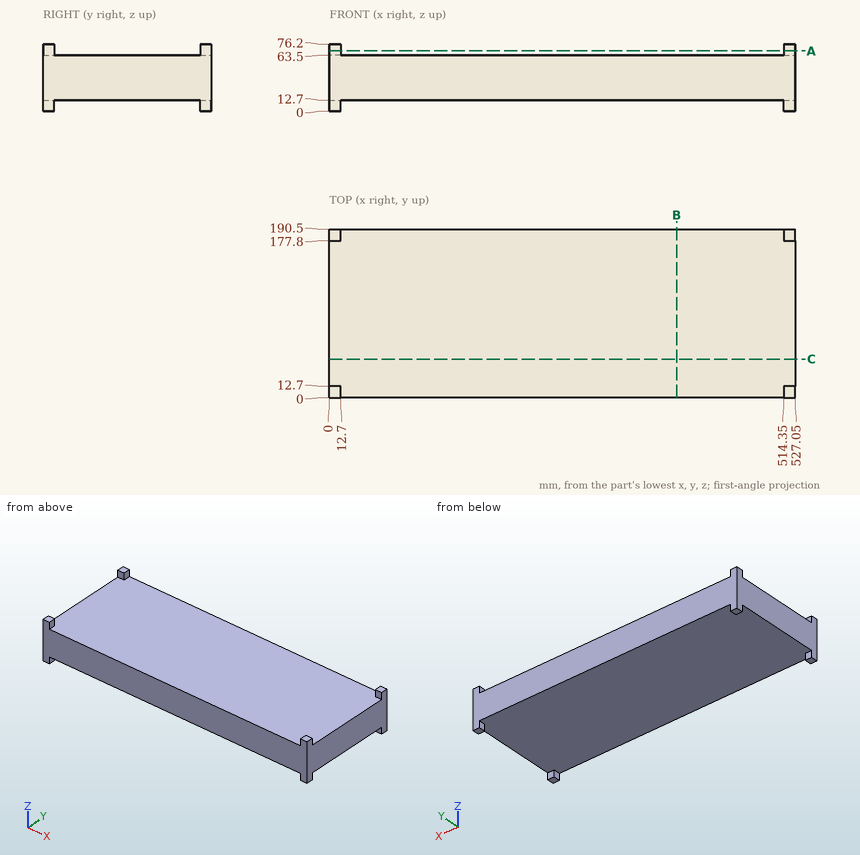
The figure shows three views and two pictorial views of one solid part (mm, origin at its lowest corner). Answer the questions. Round coordinates to 2 decimals unless told otherwise and drop trailing zeros. Write each loop counter-clockwise with the first axis right and the second up, starting at its lowest first coordinate (ties: lowest second). Pieces come first, ordered by that corner, then holes. Notation, with made-up numbers: M 76,65 L 134,65 A32 ccw 134,95 Z; hole C 85,39.25 d7. An arc over 180 degrees is marked long. Write each question's results on one line, items separated by ' | '. Start each with the question number.
(1) The part is cut by section C-C, the plane y = 43.5. Write down the section's boundary in (x, z).
(2) Each of these flat-tipped pins is pushed along its axis until it touches: P1, Ø8, axis at x = 93.5, y = 24.5, coming from the -Z side; P2, Ø1, axis at x = 90, y = 138.5, coming from the +Z side. Where does it stop, or does it pass through?
(3) The part is cut by section A-A, the plane z = 68.5. Write down the section's boundary in (x, y), and give its area (3 significant figures).
(4) The part is cut by section B-B, the plane x = 393. Write down the section's boundary in (y, z).
(5) Find the intervals of material crossed by line 1 (Z direction, x = 229, y = 169), in increasing order.
Worked answers:
1) outline: M 0,12.7 L 527.05,12.7 L 527.05,63.5 L 0,63.5 Z
2) P1: stops at z = 12.7 | P2: stops at z = 63.5
3) outline: M 0,0 L 12.7,0 L 12.7,12.7 L 0,12.7 Z; M 0,177.8 L 12.7,177.8 L 12.7,190.5 L 0,190.5 Z; M 514.35,0 L 527.05,0 L 527.05,12.7 L 514.35,12.7 Z; M 514.35,177.8 L 527.05,177.8 L 527.05,190.5 L 514.35,190.5 Z | area: 645 mm²
4) outline: M 0,12.7 L 190.5,12.7 L 190.5,63.5 L 0,63.5 Z
5) line 1: z = 12.7 to 63.5
